Design review of the part built by this model. Coordinates are the model's own, in mm. Coordinates: 2 decimals unless noted, no trailing zeros. Loops run counter-clockwise (first coordinate to the right, second up) from the corner with the lowest first, then second, coordinate; pieces in that order, holes last. Notation, with made-up numbers: (78, 68) - (133, 68) arc R34 ccw to (133, 99) - close; hole circle Ø8 at (-9, -2). An arc over 180 degrees is marked (long way). Answer in a Markdown table with one row per item. Add a question column.
(1) Clearance check with flat-ended pins moving along their axes: pin 1 (1 mm diameter, centred on y = -1.5, z = -38, fed in from -X); pin 2 (4 mm diameter, centred on x = 53.5, y = -5, fed in from -Z); pin 3 (12 mm diameter, centred on x = -23.5, z = 7, fed in from -Y); pin 4 (1.5 mm diameter, centred on y = -3.5, z = -12, fed in from +X). State where each tip first meets the part, or that it passes through.
(2) We need section C-C, the plane z = -26.5. Write out the cut boundary in (x, y), plus the area to 3 significant figures.
(3) To check wall thickness, follow L1, parallel to X at y = -3.5, z = -2.5; L2, parallel to X at y = -4.25, z = -30; L3, parallel to Z at x = -14, y = -4.25. State the ranges of each line that lie inside material, in increasing order. Write a range as [from, to].
(4) We need section D-D, the plane z = 26. Write out the cut boundary in (x, y), plus the area to 3 significant figures.
(5) We need section B-B, the plane y = -5. Write out the cut boundary in (x, z).
(6) We need section A-A, the plane z = 0. Write out the cut boundary in (x, y), plus the area to 3 significant figures.
from build123d import *

# Parameters (mm, degrees)
F0_R     = 10.5
F1_DEPTH = 7


with BuildPart() as f1:
    # F0 (on Front) → F1 (new body)
    with BuildSketch(Plane.XZ):
        with BuildLine():
            ThreePointArc((11.295326, 5.354027), (12.195113, 2.743941), (12.5, 0))
            ThreePointArc((12.5, 0), (12.452429, -1.089502), (12.310078, -2.170712))
            ThreePointArc((12.310078, -2.170712), (26.882949, -8.961501), (42.415141, -4.81007))
            ThreePointArc((42.415141, -4.81007), (42.880339, 0.767824), (45.733166, 5.583494))
            ThreePointArc((45.733166, 5.583494), (39.308861, 9.012266), (32.218698, 10.672916))
            ThreePointArc((32.218698, 10.672916), (20.823945, 11.683957), (11.295326, 5.354027))
        make_face()
        with BuildLine():
            ThreePointArc((45.733166, 5.583494), (42.880339, 0.767824), (42.415141, -4.81007))
            ThreePointArc((42.415141, -4.81007), (55.678745, -15.501888), (67.28827, -3.033646))
            ThreePointArc((67.28827, -3.033646), (59.428378, 8.573223), (45.733166, 5.583494))
        make_face()
        with Locations((54.78827, -3.033646)):
            Circle(F0_R, mode=Mode.SUBTRACT)
        with BuildLine():
            ThreePointArc((-27.702031, 36.814337), (-22.105124, 36.751551), (-17.041928, 39.137625))
            ThreePointArc((-17.041928, 39.137625), (-13.523869, 43.501909), (-12.266921, 48.964857))
            ThreePointArc((-12.266921, 48.964857), (-32.49871, 58.786742), (-27.702031, 36.814337))
        make_face()
        with Locations((-24.766921, 48.964857)):
            Circle(F0_R, mode=Mode.SUBTRACT)
        with BuildLine():
            ThreePointArc((-10.284387, 7.105026), (-7.640688, 9.892921), (-4.275147, 11.746196))
            ThreePointArc((-4.275147, 11.746196), (-5.680587, 27.762067), (-17.041928, 39.137625))
            ThreePointArc((-17.041928, 39.137625), (-22.105124, 36.751551), (-27.702031, 36.814337))
            ThreePointArc((-27.702031, 36.814337), (-27.459282, 29.53634), (-25.352365, 22.565753))
            ThreePointArc((-25.352365, 22.565753), (-20.530576, 12.192087), (-10.284387, 7.105026))
        make_face()
        with BuildLine():
            ThreePointArc((12.310078, -2.170712), (12.452429, -1.089502), (12.5, 0))
            ThreePointArc((12.5, 0), (12.195113, 2.743941), (11.295326, 5.354027))
            ThreePointArc((11.295326, 5.354027), (4.747176, 11.563491), (-4.275147, 11.746196))
            ThreePointArc((-4.275147, 11.746196), (-7.640688, 9.892921), (-10.284387, 7.105026))
            ThreePointArc((-10.284387, 7.105026), (-12.387865, -1.67057), (-8.034931, -9.575484))
            ThreePointArc((-8.034931, -9.575484), (-4.747176, -11.563491), (-1.01094, -12.459053))
            ThreePointArc((-1.01094, -12.459053), (7.640688, -9.892921), (12.310078, -2.170712))
        make_face()
        Circle(F0_R, mode=Mode.SUBTRACT)
        with BuildLine():
            ThreePointArc((-6.866333, -33.238669), (-0.293369, -23.876044), (-1.01094, -12.459053))
            ThreePointArc((-1.01094, -12.459053), (-4.747176, -11.563491), (-8.034931, -9.575484))
            ThreePointArc((-8.034931, -9.575484), (-21.202362, -18.800566), (-25.373214, -34.327555))
            ThreePointArc((-25.373214, -34.327555), (-20.775215, -37.519374), (-18.031136, -42.397831))
            ThreePointArc((-18.031136, -42.397831), (-11.849579, -38.548606), (-6.866333, -33.238669))
        make_face()
        with BuildLine():
            ThreePointArc((-18.031136, -42.397831), (-20.775215, -37.519374), (-25.373214, -34.327555))
            ThreePointArc((-25.373214, -34.327555), (-40.373926, -52.936505), (-17.521349, -45.931211))
            ThreePointArc((-17.521349, -45.931211), (-17.649452, -44.146228), (-18.031136, -42.397831))
        make_face()
        with Locations((-30.021349, -45.931211)):
            Circle(F0_R, mode=Mode.SUBTRACT)
    extrude(amount=F1_DEPTH)


solid = f1.part
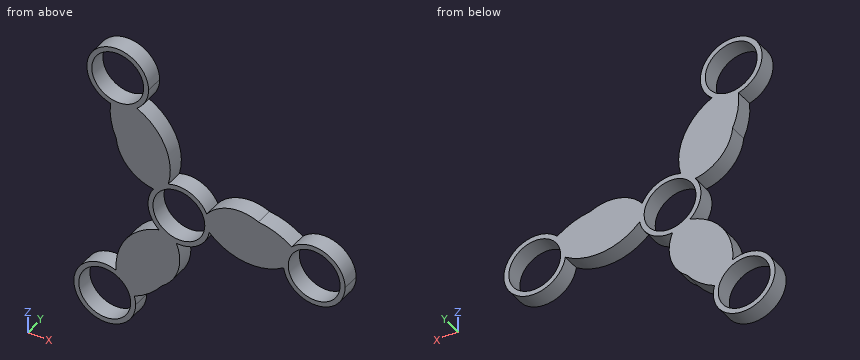
Responses:
| question | item | result |
|---|---|---|
| 1 | pin 1 | stops at x = -40.07 |
| 1 | pin 2 | stops at z = -15.53 |
| 1 | pin 3 | stops at y = -7 |
| 1 | pin 4 | stops at x = 64.21 |
| 2 | outline | (-24.73, -7) - (-1.27, -7) - (-1.27, 0) - (-24.73, 0) - close |
| 2 | area | 164 mm2 |
| 3 | L1 | x = [-12.25, -10.2], [10.2, 12.25], [12.65, 44.3], [65.27, 67.28] |
| 3 | L2 | x = [-25.35, -3.45] |
| 3 | L3 | z = [-40.15, -12.1], [7.99, 37.43], [42.61, 55.31] |
| 4 | outline | (-26.64, -7) - (-4.94, -7) - (-4.94, 0) - (-26.64, 0) - close |
| 4 | area | 152 mm2 |
| 5 | outline | (-27.7, 36.81) arc R28.07 ccw to (-25.35, 22.57) arc R17.28 ccw to (-10.28, 7.11) arc R12.5 ccw to (-8.03, -9.58) arc R23.53 ccw to (-25.37, -34.33) arc R12.5 ccw (long way) to (-17.52, -45.93) arc R12.5 ccw to (-18.03, -42.4) arc R28.07 ccw to (-6.87, -33.24) arc R17.28 ccw to (-1.01, -12.46) arc R12.5 ccw to (12.31, -2.17) arc R23.53 ccw to (42.42, -4.81) arc R12.5 ccw (long way) to (45.73, 5.58) arc R28.07 ccw to (32.22, 10.67) arc R17.28 ccw to (11.3, 5.35) arc R12.5 ccw to (-4.28, 11.75) arc R23.53 ccw to (-17.04, 39.14) arc R12.5 ccw to (-12.27, 48.96) arc R12.5 ccw (long way) to start; hole circle Ø21 at (-30.02, -45.93); hole circle Ø21 at (-24.77, 48.96); hole circle Ø21 at (0, 0); hole circle Ø21 at (54.79, -3.03) |
| 6 | outline | (-12.5, -7) - (-10.5, -7) - (-10.5, 0) - (-12.5, 0) - close; (10.5, -7) - (44.74, -7) - (44.74, 0) - (10.5, 0) - close; (64.84, -7) - (66.91, -7) - (66.91, 0) - (64.84, 0) - close |
| 6 | area | 268 mm2 |
